Source: CAD feature listing. Evaluate the final solid. Frame: model axes, mm. Coordinates: 2 decimals unless noted, no trailing zeros. Order: outer loops, then holes, each group sorted by start corner. A loop starts at its lowest first (then second) coordinate and runs counter-clockwise, first axis right, second up. Notation, with made-up numbers: (78, -16) -> (125, -16) arc R33 ccw to (125, 22) -> close; hole circle Ø2 at (80, 53.5). An arc over 180 degrees is marked (long way). Write each question's results on one line, items separated by ' | '. Start each with the question number.
Autodesk Fusion 360 part; units mm, degrees
sketch "Sketch1" plane through (0, 0, 0) normal (0, 1, 0) x (1, 0, 0) in component "WoaS Preamp Box Drilling Block"
  line L0 (33.5, -26.3) -> (-33.5, -26.3)
  line L1 (-33.5, -26.3) -> (-33.5, 26.3)
  line L2 (-33.5, 26.3) -> (33.5, 26.3)
  line L3 (33.5, 26.3) -> (33.5, -26.3)
  line L4 (33.5, -26.3) -> (-33.5, 26.3) construction
  line L5 (-33.5, -26.3) -> (33.5, 26.3) construction
  line L6 (0, 0) -> (-10.05, 0) construction
  line L7 (-10.05, 0) -> (-10.05, -17.7) construction
  line L8 (0, 0) -> (23.45, 0) construction
  line L9 (23.45, 0) -> (23.45, 17.5) construction
  circle A0 centre (23.45, 17.5) radius 2
  circle A1 centre (-10.05, -17.7) radius 2
  dimension "d1" = 67
  dimension "d2" = 52.6
  dimension "d3" = 10.05
  dimension "d4" = 17.7
  dimension "d5" = 23.45
  dimension "d6" = 17.5
  dimension "d7" = 4
  dimension "d8" = 4
sketch "Sketch2" plane through (0, 0, 0) normal (1, 0, 0) x (0, 0, -1) in component "WoaS Preamp Box Drilling Block"
  line L0 (-26.3, -20.5) -> (26.3, -20.5)
  line L1 (26.3, -20.5) -> (26.3, 20.5)
  line L2 (26.3, 20.5) -> (-26.3, 20.5)
  line L3 (-26.3, 20.5) -> (-26.3, -20.5)
  line L4 (-26.3, -20.5) -> (26.3, 20.5) construction
  line L5 (26.3, -20.5) -> (-26.3, 20.5) construction
  circle A0 centre (0, 0) radius 5
  line L6 (26.3, 20.5) -> (16.2834, 12.6924)
  circle A1 centre (16.2834, 12.6924) radius 4.15
  dimension "d9" = 52.6
  dimension "d10" = 41
  dimension "d11" = 10
  dimension "d12" = 12.7
  dimension "d13" = 8.3
extrude "Extrude1" add sketch "Sketch1" along normal mid plane 41 in component "WoaS Preamp Box Drilling Block"
extrude "Extrude2" cut sketch "Sketch2" along normal mid plane 67 contours A1 | A0 in component "WoaS Preamp Box Drilling Block"
chamfer "Chamfer1" distance 1 angle 45 6 faces at (-7.3094, 20.5, -9.2654) (-33.5, 0, 19.2) (-11.1667, 6.8333, 26.3) (-7.3094, -20.5, -9.2654) (33.5, 0, 19.2) (-11.1667, -6.8333, -26.3) in component "WoaS Preamp Box Drilling Block"
component "WoaS Preamp Box Drilling Block" placed x (1, 0, 0) y (0, 1, 0) z (0, 0, 1) at (0, 0, 0)
equation "d3 = ( 69.9 / 2 ) * 1 mm - 24.9 mm"
equation "d4 = ( 55 / 2 ) * 1 mm - 9.8 mm"
equation "d5 = ( 69.9 / 2 ) * 1 mm - 11.5 mm"
equation "d6 = ( 55 / 2 ) * 1 mm - 10 mm"
equation "d12 = ( 25.4 / 2 ) * 1 mm"
equation "d14 = ( 41 / 2 ) * 1 mm"
(1) First-contact query: P1, Ø6.5, axis at x = 23.45, z = -17.5, coming from the -Y side; P2, Ø3.5, axis at x = -10.05, z = 17.7, coming from the -Y side. Flat tips, straight axial feed; report the tip coordinate or a pass-through.
(2) Section D-D on z = 17.7. Return the cut outline in (x, y).
(3) Draft query along X for faces 1 (the cylindrical face through (23.016, 17.843, -19.452)), 2 (the cylindrical face through (-0.455, 11.446, -20.242)), 3 (the flat face through (-33.5, -5, 6)), 4 (the cylindrical face through (24.5, -4.9, -15.8)). Return one class per face: released by +X, released by -X, zero draft, split by the parting line, or undercut.
(4) Section B-B on z = 0. Return the cut outline in (x, y), then the cut area to 3 significant figures.
(5) Section C-C on x = -10.05. Return the cut outline in (y, z).
(6) Section A-A on y = 0. Return the cut outline in (x, z).
(7) Line query: L1, parallel to Y at x = -9, z = -16.5; L2, parallel to Z at x = -28, y = 13.5; L3, parallel to Z at x = 2, y = -3.5. Output: solid intervals per line, ascending.
Results list:
1) P1: stops at y = -20.5 | P2: passes through
2) outline: (-33.5, -19.5) -> (-32.5, -20.5) -> (-13.05, -20.5) -> (-12.05, -19.5) -> (-12.05, 19.5) -> (-13.05, 20.5) -> (-32.5, 20.5) -> (-33.5, 19.5) -> close; (-8.05, -19.5) -> (-7.05, -20.5) -> (32.5, -20.5) -> (33.5, -19.5) -> (33.5, 19.5) -> (32.5, 20.5) -> (-7.05, 20.5) -> (-8.05, 19.5) -> close
3) face 1: undercut | face 2: zero draft | face 3: released by -X | face 4: undercut
4) outline: (-33.5, -19.5) -> (-32.5, -20.5) -> (32.5, -20.5) -> (33.5, -19.5) -> (33.5, -6) -> (32.5, -5) -> (-32.5, -5) -> (-33.5, -6) -> close; (-33.5, 6) -> (-32.5, 5) -> (32.5, 5) -> (33.5, 6) -> (33.5, 19.5) -> (32.5, 20.5) -> (-32.5, 20.5) -> (-33.5, 19.5) -> close | area: 2,070 mm²
5) outline: (-20.5, -25.3) -> (-19.5, -26.3) -> (19.5, -26.3) -> (20.5, -25.3) -> (20.5, 14.7) -> (19.5, 15.7) -> (-19.5, 15.7) -> (-20.5, 14.7) -> close; (-20.5, 20.7) -> (-19.5, 19.7) -> (19.5, 19.7) -> (20.5, 20.7) -> (20.5, 25.3) -> (19.5, 26.3) -> (-19.5, 26.3) -> (-20.5, 25.3) -> close; hole circle Ø10 at (0, 0); hole circle Ø8.3 at (12.69, -16.28)
6) outline: (-33.5, -25.3) -> (-32.5, -26.3) -> (32.5, -26.3) -> (33.5, -25.3) -> (33.5, -6) -> (32.5, -5) -> (-32.5, -5) -> (-33.5, -6) -> close; (-33.5, 6) -> (-32.5, 5) -> (32.5, 5) -> (33.5, 6) -> (33.5, 25.3) -> (32.5, 26.3) -> (-32.5, 26.3) -> (-33.5, 25.3) -> close; hole circle Ø4 at (-10.05, 17.7); hole circle Ø4 at (23.45, -17.5)
7) L1: y = -20.5 to 8.55, 16.84 to 20.5 | L2: z = -26.3 to -20.35, -12.21 to 26.3 | L3: z = -26.3 to -3.57, 3.57 to 26.3
